Check sheet for the modelled part. Datum: model origin and axes. Units: mm. Face numbers are marked on the shaded views. A direction names the side the tool comes from. Round coordinates to 2 decimals unless told otherwise and drop trailing zeros. Write each loop counter-clockwise with the first axis right and the second up, starting at its lowest first coordinate (ties: lowest second). Pieces come first, ordered by that corner, then holes.
Item 1: Cross-section at C-C on x = -14. Enter the section's corners in (y, z), plus the area to 3 significant figures.
Item 2: Cross-section at A-A on y = 7.5. Enter the section's corners in (x, z).
Item 3: Go/stop test with flat-tipped pins: pin 1 Ø2 at (y, z) = (-9.5, 13.5) entering from +X; pin 2 Ø4 at (x, y) = (-6.5, -9) entering from +Z. Record where each tip stops, or that it passes through.
Item 4: Cross-section at D-D on y = -14. Enter the section's corners in (x, z).
Item 5: Material ranges on line 1 (Z direction, x = -19.5, y = 15); line 2 (Y direction, x = 22, z = 17); line 3 (Y direction, x = 14, z = 17.5), recorded low to high.
Item 6: Cross-section at B-B on x = 15.5. Enter the section's corners in (y, z), plus the area to 3 significant figures.
Item 7: Tool access check on the marked faces 1 and 2. Record the directions out of +Z, -Z, +X, -X, +Y, -Y that give a thin tool (end or side, any length) a straight path to the whole face; none if there is none.
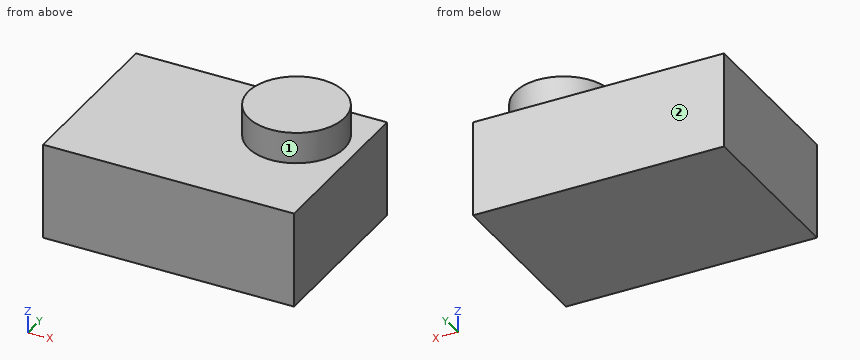
from build123d import *

# Parameters (mm, degrees)
SKETCH_1_W      = 60
SKETCH_1_H      = 42
SKETCH_1_R      = 11.5
EXTRUDE_1_DEPTH = 11.5
EXTRUDE_START   = 11.5
SKETCH_1_3_R    = 11.5
EXTRUDE_2_DEPTH = 7.5


with BuildPart() as part:
    # Эскиз1 → Бобышка-Вытянуть1 (new, symmetric)
    with BuildSketch(Plane.XY):
        Rectangle(SKETCH_1_W, SKETCH_1_H)
        with Locations((15.5, 7.5)):
            Circle(SKETCH_1_R, mode=Mode.SUBTRACT)
        with Locations((15.5, 7.5)):
            Circle(SKETCH_1_R)
    extrude(amount=EXTRUDE_1_DEPTH, both=True)

    # Эскиз1<3> → Бобышка-Вытянуть2 (add)
    with BuildSketch(Plane.XY.offset(EXTRUDE_START)):
        with Locations((15.5, 7.5)):
            Circle(SKETCH_1_3_R)
    extrude(amount=EXTRUDE_2_DEPTH)


solid = part.part
Response values:
1. outline: (-21, -11.5) - (21, -11.5) - (21, 11.5) - (-21, 11.5) - close
1. area: 966 mm2
2. outline: (-30, -11.5) - (30, -11.5) - (30, 11.5) - (27, 11.5) - (27, 19) - (4, 19) - (4, 11.5) - (-30, 11.5) - close
3. pin 1: passes through
3. pin 2: stops at z = 11.5
4. outline: (-30, -11.5) - (30, -11.5) - (30, 11.5) - (-30, 11.5) - close
5. line 1: z = -11.5 to 11.5
5. line 2: y = -1.99 to 16.99
5. line 3: y = -3.9 to 18.9
6. outline: (-21, -11.5) - (21, -11.5) - (21, 11.5) - (19, 11.5) - (19, 19) - (-4, 19) - (-4, 11.5) - (-21, 11.5) - close
6. area: 1,140 mm2
7. face 1: +Z
7. face 2: +Z, -Z, +X, -X, +Y
